```python
from build123d import *

# Parameters (mm, degrees)
SKETCH_1_W             = 112
SKETCH_1_H             = 110.77381068
SKETCH_1_R             = 5.25
SM_BASE_FLANGE_1_DEPTH = 5
CHAMFER_1_SIZE         = 15
CUT_EXTRUDE_1_DEPTH    = 10


# Sheet-metal steps are written as plain solids
with BuildPart() as part:
    # Sketch 1 → Базовая кромка1 (new body)
    with BuildSketch(Plane.XY):
        with Locations((0, 58.38690534)):
            Rectangle(SKETCH_1_W, SKETCH_1_H)
        with Locations((-28, 43)):
            Circle(SKETCH_1_R, mode=Mode.SUBTRACT)
        with Locations(Location((28, 73.77381068, 0), (0, 0, 180))):
            Circle(SKETCH_1_R, mode=Mode.SUBTRACT)
        with Locations(Location((28, 43, 0), (0, 0, 180))):
            Circle(SKETCH_1_R, mode=Mode.SUBTRACT)
    extrude(amount=-SM_BASE_FLANGE_1_DEPTH)

    # Фаска1
    chamfer_1_edges = [part.edges().sort_by_distance(p)[0] for p in [
        (56, 3, -2.5),
        (-56, 3, -2.5),
        (-56, 113.77381068, -2.5),
        (56, 113.77381068, -2.5),
    ]]
    chamfer(chamfer_1_edges, length=CHAMFER_1_SIZE)

    # Sketch 2 → Вырез-Вытянуть1 (cut)
    with BuildSketch(Plane.XY):
        Polygon((-56, 113.77381068), (-56, 86.768448621), (-6.468509112, 113.77381068), align=None)
    extrude(amount=-CUT_EXTRUDE_1_DEPTH, mode=Mode.SUBTRACT)


solid = part.part
```
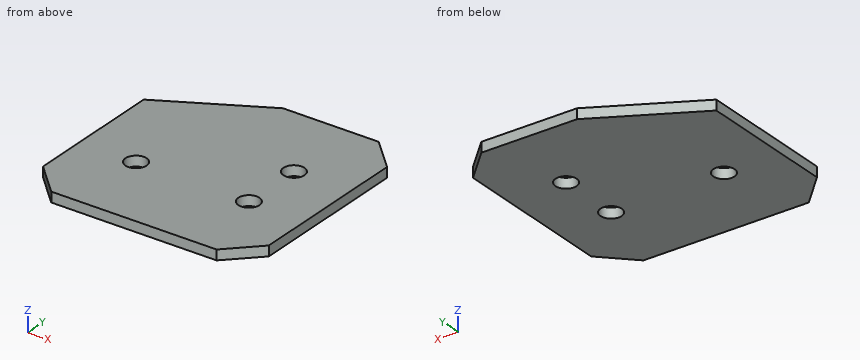
Here's how the part is built. I have some questions about the finished solid (model axes, mm). Round coordinates to 2 decimals unless told otherwise and drop trailing zeros. Loops run counter-clockwise (first coordinate to the right, second up) from the corner with the lowest first, then second, coordinate; pieces in that order, holes last. Notation, with made-up numbers: (25.5, -7) -> (75.5, -7) arc R20 ccw to (75.5, 27) -> close; hole circle Ø1 at (62.25, -22.5). An arc over 180 degrees is marked (long way). Answer as CSV lines item,"result". Start each with the question number.
1. Imagine slicing it at C-C on y = 72. Write out the boundary of the cut face in (x, z), plus the area to 3 significant figures.
2. I need wall thicknesses on probe 1 along Y at (x, z) = (28, -2.8); probe 2 along Y at (x, z) = (-26, -4.15); probe 3 along Y at (x, z) = (-28, -1.4). Which ranges of each line are inside material? Lowest first, please. Write a range as from..to.
3. I'm going to push a flat-ended pin straight in: P1, Ø13.5, axis at x = 28, y = 73.77, coming from the +Z side. Where does the tip first touch, or does it pass through?
4. Imagine slicing it at B-B on x = 28. Write out the boundary of the cut face in (y, z).
5. Imagine slicing it at D-D on x = -28. Write out the boundary of the cut face in (y, z), plus the area to 3 significant figures.
6. Imagine slicing it at A-A on y = 43. Write out the boundary of the cut face in (x, z), plus the area to 3 significant figures.
Solution:
1,outline,"(-56, -5) -> (23.06, -5) -> (23.06, 0) -> (-56, 0) -> close; (32.94, -5) -> (56, -5) -> (56, 0) -> (32.94, 0) -> close"
1,area,"511 mm²"
2,probe 1,"3..37.75, 48.25..68.52, 79.02..113.77"
2,probe 2,"3..38.15, 47.85..103.12"
2,probe 3,"3..37.75, 48.25..102.03"
3,P1,"z = 0"
4,outline,"(3, -5) -> (37.75, -5) -> (37.75, 0) -> (3, 0) -> close; (48.25, -5) -> (68.52, -5) -> (68.52, 0) -> (48.25, 0) -> close; (79.02, -5) -> (113.77, -5) -> (113.77, 0) -> (79.02, 0) -> close"
5,outline,"(3, -5) -> (37.75, -5) -> (37.75, 0) -> (3, 0) -> close; (48.25, -5) -> (102.03, -5) -> (102.03, 0) -> (48.25, 0) -> close"
5,area,"443 mm²"
6,outline,"(-56, -5) -> (-33.25, -5) -> (-33.25, 0) -> (-56, 0) -> close; (-22.75, -5) -> (22.75, -5) -> (22.75, 0) -> (-22.75, 0) -> close; (33.25, -5) -> (56, -5) -> (56, 0) -> (33.25, 0) -> close"
6,area,"455 mm²"
